from build123d import *

# Parameters (mm, degrees)
BOSS_EXTRUDE1_DEPTH = 500
FILLET1_R           = 50
SHELL1_START        = 25.4
SHELL1_DEPTH        = 449.2
SHELL1_START_2      = 24
SHELL1_2_DEPTH      = 452
SHELL1_START_3      = 154
SHELL1_3_DEPTH      = 20.6
SHELL1_START_4      = 174.6
SHELL1_4_DEPTH      = 500.4


with BuildPart() as part:
    # Sketch1 → Boss-Extrude1 (new body)
    with BuildSketch(Plane(origin=(0, 0, 0), x_dir=(0, 0, -1), z_dir=(1, 0, 0))):
        Polygon((0, 0), (-500, 0), (-500, 200), (-70, 200), (-70, 700), (0, 700), (0, 41.235294118), align=None)
    extrude(amount=BOSS_EXTRUDE1_DEPTH)

    # Fillet1
    fillet1_edges = [part.edges().sort_by_distance(p)[0] for p in [
        (250, 200, 500),
        (250, 700, 70),
        (500, 450, 70),
        (500, 200, 285),
        (0, 200, 285),
        (0, 450, 70),
    ]]
    fillet(fillet1_edges, radius=FILLET1_R)

    # Shell1: read off the stored shape, not the designer's step
    # Shell1 outline → Shell1 (cut)
    with BuildSketch(Plane.YZ.offset(SHELL1_START)):
        with BuildLine():
            Line((25.4, 25.4), (674, 25.4))
            ThreePointArc((674, 25.4), (665.36749817, 39.209372712), (650, 44.6))
            Line((650, 44.6), (174.6, 44.6))
            Line((174.6, 44.6), (174.6, 450))
            ThreePointArc((174.6, 450), (167.394826817, 467.394826817), (150, 474.6))
            Line((150, 474.6), (25.4, 474.6))
            Line((25.4, 474.6), (25.4, 25.4))
        make_face()
    extrude(amount=SHELL1_DEPTH, mode=Mode.SUBTRACT)

    # Shell1 2 outline → Shell1 2 (add)
    with BuildSketch(Plane.XY.offset(SHELL1_START_2)):
        with BuildLine():
            ThreePointArc((25.4, 150), (32.605173183, 167.394826817), (50, 174.6))
            Line((50, 174.6), (25.4, 174.6))
            Line((25.4, 174.6), (25.4, 150))
        make_face()
        with BuildLine():
            ThreePointArc((450, 174.6), (467.394826817, 167.394826817), (474.6, 150))
            Line((474.6, 150), (474.6, 174.6))
            Line((474.6, 174.6), (450, 174.6))
        make_face()
    extrude(amount=SHELL1_2_DEPTH)

    # Shell1 3 outline → Shell1 3 (cut)
    with BuildSketch(Plane(origin=(0, 0, 0), x_dir=(1, 0, 0), z_dir=(0, 1, 0)).offset(SHELL1_START_3)):
        with BuildLine():
            ThreePointArc((450, -44.6), (465.36749817, -39.209372712), (474, -25.4))
            Line((474, -25.4), (26, -25.4))
            ThreePointArc((26, -25.4), (34.63250183, -39.209372712), (50, -44.6))
            Line((50, -44.6), (450, -44.6))
        make_face()
    extrude(amount=SHELL1_3_DEPTH, mode=Mode.SUBTRACT)

    # Shell1 4 outline → Shell1 4 (add)
    with BuildSketch(Plane(origin=(0, 0, 0), x_dir=(1, 0, 0), z_dir=(0, 1, 0)).offset(SHELL1_START_4)):
        with BuildLine():
            Line((474.6, -25.4), (474, -25.4))
            ThreePointArc((474, -25.4), (465.36749817, -39.209372712), (450, -44.6))
            Line((450, -44.6), (474.6, -44.6))
            Line((474.6, -44.6), (474.6, -25.4))
        make_face()
        with BuildLine():
            ThreePointArc((50, -44.6), (34.63250183, -39.209372712), (26, -25.4))
            Line((26, -25.4), (25.4, -25.4))
            Line((25.4, -25.4), (25.4, -44.6))
            Line((25.4, -44.6), (50, -44.6))
        make_face()
    extrude(amount=SHELL1_4_DEPTH)


solid = part.part
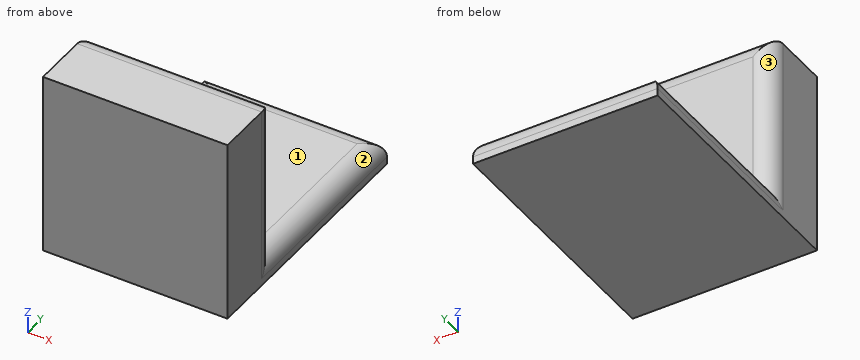
Source: CAD feature listing. Evaluate the final solid. Frame: model axes, mm. Face numbers are marked on the shaded views. A direction names the side the tool comes from. Give positions to 0.01 mm unless a question says otherwise; leave off trailing zeros. Write each loop counter-clockwise with the first axis right and the second up, starting at its lowest first coordinate (ties: lowest second). Pieces come first, ordered by that corner, then holes. Notation, with made-up numbers: M 36,47 L 92,47 A26 cw 92,75 Z; hole C 87.5,48.25 d7. An arc over 180 degrees is marked long. Return JSON: item names as keys, results as strings. Group by question number.
1) Cut plane B-B, the plane x = 113.5. Output: boundary loops of the cut face in (y, z).
2) Material intervals for line 1 along Y through (x, z) = (174, 312); line 2 along Z through (x, y) = (113.5, 394.5); line 3 along Z through (x, y) = (41.5, 43), sorted ascending. Write a range as [from, to].
3) Cut plane A-A, the plane y = 276. Output: boundary loops of the cut face in (x, z), plus the area to 3 significant figures.
4) Cut plane D-D, the plane y = 63. Output: boundary loops of the cut face in (x, z).
5) Pin query (flat end, axial travel): P1, Ø5, axis at x = 332.5, y = 171, coming from the +Z side; P2, Ø12, axis at x = 309, z = 253.5, coming from the +Y side. Return the tip coordinate at first contact, or that it passes through.
6) Cut plane C-C, the plane z = 147. Output: boundary loops of the cut face in (x, y).
7) Set-up query: the marked faces 1, 2 and 3. Return all of +Z, -Z, +X, -X, +Y, -Y with unobstructed straight access to the full face (end or side cutting, diameter ignored); none if empty.
Recorded:
{
 "1": {"outline": "M 0,0 L 700,0 L 700,20 A50 ccw 650,70 L 200,70 L 200,450 A50 ccw 150,500 L 0,500 Z; hole M 25.4,25.4 L 674,25.4 A24.6 ccw 650,44.6 L 174.6,44.6 L 174.6,450 A24.6 ccw 150,474.6 L 25.4,474.6 Z"},
 "2": {"line 1": "y = [0, 25.4], [174.6, 200]", "line 2": "z = [0, 25.4], [44.6, 70]", "line 3": "z = [0, 25.4], [474.6, 500]"},
 "3": {"outline": "M 0,0 L 500,0 L 500,20 A50 ccw 450,70 L 50,70 A50 ccw 0,20 Z; hole M 26,25.4 L 474,25.4 A24.6 ccw 450,44.6 L 50,44.6 A24.6 ccw Z", "area": "25,600 mm²"},
 "4": {"outline": "M 0,0 L 500,0 L 500,500 L 0,500 Z; hole M 25.4,25.4 L 474.6,25.4 L 474.6,474.6 L 25.4,474.6 Z"},
 "5": {"P1": "stops at z = 496.45", "P2": "stops at y = 200"},
 "6": {"outline": "M 0,0 L 500,0 L 500,150 A50 ccw 450,200 L 50,200 A50 ccw 0,150 Z; hole M 25.4,25.4 L 474.6,25.4 L 474.6,150 A24.6 ccw 450,174.6 L 50,174.6 A24.6 ccw 25.4,150 Z"},
 "7": {"face 1": "+Z, +X, -X, +Y", "face 2": "+Z, +X, +Y", "face 3": "+Z, -X, +Y"}
}
